Work out the finished part from the listing and answer in its coordinate system (mm). A direction names the side the tool comes from. Round coordinates to 2 decimals unless told otherwise and drop trailing zeros. Order: outer loops, then holes, each group sorted by start corner. A loop starts at its lowest first (then second) coordinate and runs counter-clockwise, first axis right, second up. Notation, with made-up numbers: M -3.75,35 L 35.25,35 A16 cw 35.25,63 Z; hole C 88.5,83 d3. An arc over 180 degrees is marked long. Return JSON: item names as keys, results as strings.
from build123d import *

# Parameters (mm, degrees)
STEM_START                  = 16.223730914
STEM_SERVO_SIDE_OUTLINE_W   = 12.827
STEM_SERVO_SIDE_OUTLINE_H   = 3.302
STEM_SERVO_SIDE_OUTLINE_R   = 1.5875
STEM_SERVO_SIDE_OUTLINE_W_2 = 13.335
STEM_SERVO_SIDE_OUTLINE_H_2 = 29
STEM_SERVO_SIDE_DEPTH       = 3.175
SKETCH1_R                   = 3.81
CUT_EXTRUDE1_DEPTH          = 3.175
FILLET1_R                   = 8.89
FILLET2_R                   = 8.89


# Read off the part's stored shape, not the designer's step: Stem Servo Side
with BuildPart() as part:
    # Stem Servo Side outline → Stem Servo Side (new body)
    with BuildSketch(Plane(origin=(0, 0, 0), x_dir=(1, 0, 0), z_dir=(0, 1, 0)).offset(STEM_START)):
        with BuildLine():
            Line((-2.093063075, 47.682601639), (-3.363063075, 47.682601639))
            ThreePointArc((-3.363063075, 47.682601639), (-9.64924236, 45.078780923), (-12.253063075, 38.792601639))
            Line((-12.253063075, 38.792601639), (-12.253063075, -28.517398361))
            Line((-12.253063075, -28.517398361), (6.796936925, -28.517398361))
            Line((6.796936925, -28.517398361), (6.796936925, 38.792601639))
            ThreePointArc((6.796936925, 38.792601639), (4.19311621, 45.078780924), (-2.093063075, 47.682601639))
        make_face()
        with Locations((-2.728063075, 1.581601639)):
            Rectangle(STEM_SERVO_SIDE_OUTLINE_W, STEM_SERVO_SIDE_OUTLINE_H, mode=Mode.SUBTRACT)
        with Locations((-2.728063075, 6.302601639)):
            Circle(STEM_SERVO_SIDE_OUTLINE_R, mode=Mode.SUBTRACT)
        with Locations((-2.728063075, 24.082601639)):
            Rectangle(STEM_SERVO_SIDE_OUTLINE_W_2, STEM_SERVO_SIDE_OUTLINE_H_2, mode=Mode.SUBTRACT)
        with Locations((-2.728063075, 41.862601639)):
            Circle(STEM_SERVO_SIDE_OUTLINE_R, mode=Mode.SUBTRACT)
    extrude(amount=STEM_SERVO_SIDE_DEPTH)

    # Sketch1 → Cut-Extrude1 (cut)
    with BuildSketch(Plane(origin=(0, 19.398730914, 0), x_dir=(1, 0, 0), z_dir=(0, 1, 0))):
        with Locations(Location((-2.728063075, -14.547398361, 0), (0, 0, 270))):
            Circle(SKETCH1_R)
    extrude(amount=-CUT_EXTRUDE1_DEPTH, mode=Mode.SUBTRACT)

    # Fillet1
    fillet1_edges = [part.edges().sort_by_distance(p)[0] for p in [
        (6.796936925, 17.811230914, 28.517398361),
    ]]
    fillet(fillet1_edges, radius=FILLET1_R)

    # Fillet2
    fillet2_edges = [part.edges().sort_by_distance(p)[0] for p in [
        (-12.253063075, 17.811230914, 28.517398361),
    ]]
    fillet(fillet2_edges, radius=FILLET2_R)


solid = part.part
Item 1: Which of the six approach directions +Z, -Z, +X, -X, +Y, -Y give full straight-line access (tool end or side, diameter ignored) to faces 5 (the cylindrical face through (-9.58, 17.83, 25.98)), 6 (the flat face through (3.685, 18, -2))?
Output:
{"face 5": "+Z, -X, +Y, -Y", "face 6": "+Y, -Y"}
Item 2: Find section C-C (y = 16.85). Determine the outline of the cut face in (x, z) (1 decimal), plus the area to 3 significant figures.
Output:
{"outline": "M -12.3,-38.8 A8.9 ccw -3.4,-47.7 L -2.1,-47.7 A8.9 ccw 6.8,-38.8 L 6.8,19.6 A8.9 ccw -2.1,28.5 L -3.4,28.5 A8.9 ccw -12.3,19.6 Z; hole M -9.4,-38.6 L 3.9,-38.6 L 3.9,-9.6 L -9.4,-9.6 Z; hole M -9.1,-3.2 L 3.7,-3.2 L 3.7,0.1 L -9.1,0.1 Z; hole C -2.7,14.5 d7.6; hole C -2.7,-41.9 d3.2; hole C -2.7,-6.3 d3.2", "area": "893 mm^2"}
Item 3: Find section A-A (z = -2). Determine the outline of the cut face in (x, y).
Output:
{"outline": "M -12.25,16.22 L -9.14,16.22 L -9.14,19.4 L -12.25,19.4 Z; M 3.69,16.22 L 6.8,16.22 L 6.8,19.4 L 3.69,19.4 Z"}
Item 4: Find section D-D (z = 12). Determine the outline of the cut face in (x, y), plus the area to 3 significant figures.
Output:
{"outline": "M -12.25,16.22 L -5.56,16.22 L -5.56,19.4 L -12.25,19.4 Z; M 0.11,16.22 L 6.8,16.22 L 6.8,19.4 L 0.11,19.4 Z", "area": "42.5 mm^2"}
Item 5: Each of these flat-tipped pins is pushed along its axis until it touches: pin 1 (1.6 mm diameter, centred on x = -5.5, y = 18, fed in from +Z); pin 2 (1 mm diameter, centred on x = -0.5, y = 18.5, fed in from -Z); pin 3 (1 mm diameter, centred on x = -5.5, y = 18, fed in from -Z). Where does it stop, or does it pass through?
Output:
{"pin 1": "stops at z = 28.42", "pin 2": "stops at z = -47.62", "pin 3": "stops at z = -47.53"}
Item 6: Consider line 1 along X through (y, z) = (17.5, -34); line 2 along Z through (x, y) = (-2.5, 17.35); line 3 along Z through (x, y) = (1.75, 17.25). Determine where each line is inside the solid, lowest interval first. Write a range as [from, to].
Output:
{"line 1": "x = [-12.25, -9.4], [3.94, 6.8]", "line 2": "z = [-47.68, -43.43], [-40.29, -38.58], [-9.58, -7.87], [-4.73, -3.23], [0.07, 10.74], [18.35, 28.52]", "line 3": "z = [-46.81, -38.58], [-9.58, -3.23], [0.07, 27.64]"}
Item 7: The mould has two halves that part along Z. Classify faces 1 (the cylindrical face through (-3.072, 17.789, -40.313)), 2 (the cylindrical face through (-9.58, 17.79, -45.15)), 3 (the flat face through (6, 19.399, -2)), 4 (the cylindrical face through (4.262, 17.833, 25.844)): pulls with the +Z half, pulls with the -Z half, needs draft (parallel to the pull), parting line crosses it, or undercut.
Output:
{"face 1": "undercut", "face 2": "pulls with the -Z half", "face 3": "needs draft", "face 4": "pulls with the +Z half"}
Item 8: Find section B-B (x = 3). Determine the outline of the cut face in (y, z).
Output:
{"outline": "M 16.22,-46.08 L 19.4,-46.08 L 19.4,-38.58 L 16.22,-38.58 Z; M 16.22,-9.58 L 19.4,-9.58 L 19.4,-3.23 L 16.22,-3.23 Z; M 16.22,0.07 L 19.4,0.07 L 19.4,26.91 L 16.22,26.91 Z"}
